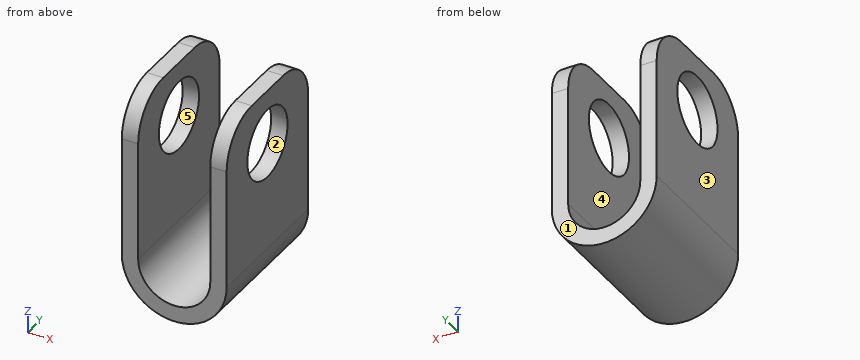
```python
from build123d import *

# Parameters (mm, degrees)
F1_DEPTH      = 8.255
F2_R          = 5.08
F3_R          = 4.064
F4_DEPTH      = 6.097
F4_DEPTH_BACK = 6.097


with BuildPart() as f1:
    # F0 (on Front) → F1 (new body, symmetric)
    with BuildSketch(Plane.XZ):
        with BuildLine():
            ThreePointArc((4.191, 0), (0, -4.191), (-4.191, 0))
            Line((-4.191, 0), (-4.191, 19.05))
            Line((-4.191, 19.05), (-6.096, 19.05))
            Line((-6.096, 19.05), (-6.096, 0))
            ThreePointArc((-6.096, 0), (0, -6.096), (6.096, 0))
            Line((6.096, 0), (6.096, 19.05))
            Line((6.096, 19.05), (4.191, 19.05))
            Line((4.191, 19.05), (4.191, 0))
        make_face()
    extrude(amount=F1_DEPTH, both=True)

    # F2
    f2_edges = [f1.edges().sort_by_distance(p)[0] for p in [
        (5.1435, -8.255, 19.05),
        (5.1435, 8.255, 19.05),
        (-5.1435, 8.255, 19.05),
        (-5.1435, -8.255, 19.05),
    ]]
    fillet(f2_edges, radius=F2_R)

    # F3 (on Right) → F4 (cut, two sides)
    with BuildSketch(Plane.YZ) as f4_sk:
        with Locations((0, 12.7)):
            Circle(F3_R)
    extrude(amount=F4_DEPTH, mode=Mode.SUBTRACT)
    extrude(f4_sk.sketch, amount=-F4_DEPTH_BACK, mode=Mode.SUBTRACT)


solid = f1.part
```
Can you work these out from the model? Positions are in its coordinate system, mm. Face numbers are marked on the shaded views. A direction names the side the tool comes from. Give positions to 0.01 mm unless a question says otherwise; leave off trailing zeros. Loops run counter-clockwise (first coordinate to the right, second up) from the corner with the lowest first, then second, coordinate; pieces in that order, holes last. Notation, with made-up numbers: M -4,53.25 L 7,53.25 A3 ccw 7,58.25 Z; hole C -28.5,29 d8. An arc over 180 degrees is marked long. One line per item, written item: value.
(1) Suppose I cut it at D-D on x = -5. List the corners of the cut face in (y, z) for me (3 decimals), plus the area to 3 significant figures.
Returned:
outline: M -8.255,-3.487 L 8.255,-3.487 L 8.255,13.97 A5.08 ccw 3.175,19.05 L -3.175,19.05 A5.08 ccw -8.255,13.97 Z; hole C 0,12.7 d8.128
area: 309 mm^2
(2) Suppose I cut it at A-A on z = 12.7. List the corners of the cut face in (x, y) for me (3 decimals), plus the area to 3 significant figures.
Returned:
outline: M -6.096,-8.255 L -4.191,-8.255 L -4.191,-4.064 L -6.096,-4.064 Z; M -6.096,4.064 L -4.191,4.064 L -4.191,8.255 L -6.096,8.255 Z; M 4.191,-8.255 L 6.096,-8.255 L 6.096,-4.064 L 4.191,-4.064 Z; M 4.191,4.064 L 6.096,4.064 L 6.096,8.255 L 4.191,8.255 Z
area: 31.9 mm^2
(3) Suppose I cut it at C-C on z = 2.75. List the corners of the cut face in (x, y) for me (3 decimals), plus the area to 3 significant figures.
Returned:
outline: M -6.096,-8.255 L -4.191,-8.255 L -4.191,8.255 L -6.096,8.255 Z; M 4.191,-8.255 L 6.096,-8.255 L 6.096,8.255 L 4.191,8.255 Z
area: 62.9 mm^2
(4) Will these pins go through, and if not, where does the flat tip stop? pin 1 (3 mm diameter, centred on x = -3.5, y = -4, fed in from +Z); pin 2 (3 mm diameter, centred on x = -2.5, y = -6.5, fed in from -Z); pin 3 (3 mm diameter, centred on x = 1.5, z = 0, fed in from +Y); pin 4 (6 mm diameter, centred on x = -0.5, y = 2, fed in from +Z).
Returned:
pin 1: z = 19.05
pin 2: z = -6.01
pin 3: through
pin 4: z = -2.31
(5) Which directions (+Z, -Z, +X, -X, +Y, -Y) give clear straight access to the entire face, cutting with the end or side of a thin tool? Please do the marked faces 4 and 5.
Returned:
face 4: +Z, +Y, -Y
face 5: +X, -X
(6) Suppose I cut it at B-B on y = 0. List the corners of the cut face in (x, z) for me.
Returned:
outline: M -6.1,0 A6.1 ccw 6.1,0 L 6.1,8.64 L 4.19,8.64 L 4.19,0 A4.19 cw -4.19,0 L -4.19,8.64 L -6.1,8.64 Z; M -6.1,16.76 L -4.19,16.76 L -4.19,19.05 L -6.1,19.05 Z; M 4.19,16.76 L 6.1,16.76 L 6.1,19.05 L 4.19,19.05 Z
(7) We'd pull the mould along Y, two halves only. Please class the marked faces 1, 2 and 3: released by +Y, released by -Y, zero draft, split by the parting line, or undercut.
Returned:
face 1: released by +Y
face 2: undercut
face 3: zero draft
(8) I need wall thicknesses on line 1 (X direction, y = 5, z = 13); line 2 (Y direction, x = 4.6, z = 12.7) (3 decimals); line 3 (X direction, y = 2.25, z = -1). Which ranges of each line are inside material? Lowest first, please.
Returned:
line 1: -6.1 to -4.19, 4.19 to 6.1
line 2: -8.255 to -4.064, 4.064 to 8.255
line 3: -6.01 to -4.07, 4.07 to 6.01
